```python
from build123d import *

# Parameters (mm, degrees)
SKETCH_1_R          = 1.55
SKETCH_1_R_2        = 6
EXTRUDE_1_DEPTH     = 7
CUT_EXTRUDE_START   = -2
CUT_EXTRUDE_3_DEPTH = 2
SKETCH_4_R          = 2.5
CUT_EXTRUDE_4_DEPTH = 3
CUT_EXTRUDE_5_DEPTH = 5
CUT_EXTRUDE_6_DEPTH = 2
SKETCH_7_W          = 5
SKETCH_7_H          = 3
CUT_EXTRUDE_7_DEPTH = 2


with BuildPart() as part:
    # 草图1 → 凸台-拉伸1 (new body)
    with BuildSketch(Plane.XY):
        with BuildLine():
            Line((0, 3), (73.66, 3))
            Line((73.66, 3), (133.66, 3))
            ThreePointArc((133.66, 3), (135.781320344, 2.121320344), (136.66, 0))
            Line((136.66, 0), (136.66, -21.844))
            Line((136.66, -21.844), (136.66, -43.688))
            ThreePointArc((136.66, -43.688), (135.781320344, -45.809320344), (133.66, -46.688))
            Line((133.66, -46.688), (73.66, -46.688))
            Line((73.66, -46.688), (0, -46.688))
            ThreePointArc((0, -46.688), (-2.121320344, -45.809320344), (-3, -43.688))
            Line((-3, -43.688), (-3, 0))
            ThreePointArc((-3, 0), (-2.121320344, 2.121320344), (0, 3))
        make_face()
        Circle(SKETCH_1_R, mode=Mode.SUBTRACT)
        with Locations((73.66, 0)):
            Circle(SKETCH_1_R, mode=Mode.SUBTRACT)
        with Locations((0, -43.688)):
            Circle(SKETCH_1_R, mode=Mode.SUBTRACT)
        with Locations((73.66, -43.688)):
            Circle(SKETCH_1_R, mode=Mode.SUBTRACT)
        with Locations((106.66, -21.844)):
            Circle(SKETCH_1_R_2, mode=Mode.SUBTRACT)
        with Locations((91.16, -6.344)):
            Circle(SKETCH_1_R, mode=Mode.SUBTRACT)
        with Locations(Location((91.16, -37.344, 0), (0, 0, 180))):
            Circle(SKETCH_1_R, mode=Mode.SUBTRACT)
        with Locations((122.16, -37.344)):
            Circle(SKETCH_1_R, mode=Mode.SUBTRACT)
        with Locations(Location((122.16, -6.344, 0), (0, 0, 180))):
            Circle(SKETCH_1_R, mode=Mode.SUBTRACT)
        with Locations((99.942485579, -15.126485579)):
            Circle(SKETCH_1_R, mode=Mode.SUBTRACT)
        with Locations((113.377514421, -15.126485579)):
            Circle(SKETCH_1_R, mode=Mode.SUBTRACT)
        with Locations((113.377514421, -28.561514421)):
            Circle(SKETCH_1_R, mode=Mode.SUBTRACT)
        with Locations((99.942485579, -28.561514421)):
            Circle(SKETCH_1_R, mode=Mode.SUBTRACT)
        with BuildLine():
            Line((11.83, -15.844), (11.83, -4.844))
            ThreePointArc((11.83, -4.844), (12.708679656, -2.722679656), (14.83, -1.844))
            Line((14.83, -1.844), (36.83, -1.844))
            Line((36.83, -1.844), (58.83, -1.844))
            ThreePointArc((58.83, -1.844), (60.951320344, -2.722679656), (61.83, -4.844))
            Line((61.83, -4.844), (61.83, -15.844))
            ThreePointArc((61.83, -15.844), (60.951320344, -17.965320344), (58.83, -18.844))
            Line((58.83, -18.844), (36.83, -18.844))
            Line((36.83, -18.844), (14.83, -18.844))
            ThreePointArc((14.83, -18.844), (12.708679656, -17.965320344), (11.83, -15.844))
        make_face(mode=Mode.SUBTRACT)
        with BuildLine():
            Line((36.83, -41.844), (58.83, -41.844))
            ThreePointArc((58.83, -41.844), (60.951320344, -40.965320344), (61.83, -38.844))
            Line((61.83, -38.844), (61.83, -27.844))
            ThreePointArc((61.83, -27.844), (60.951320344, -25.722679656), (58.83, -24.844))
            Line((58.83, -24.844), (36.83, -24.844))
            Line((36.83, -24.844), (14.83, -24.844))
            ThreePointArc((14.83, -24.844), (12.708679656, -25.722679656), (11.83, -27.844))
            Line((11.83, -27.844), (11.83, -38.844))
            ThreePointArc((11.83, -38.844), (12.708679656, -40.965320344), (14.83, -41.844))
            Line((14.83, -41.844), (36.83, -41.844))
        make_face(mode=Mode.SUBTRACT)
    extrude(amount=EXTRUDE_1_DEPTH)

    # 草图2 → 切除-拉伸3 (cut)
    with BuildSketch(Plane.XY.offset(7).offset(CUT_EXTRUDE_START)):
        with BuildLine():
            Line((1.933137513, -8), (11.83, -8))
            Line((11.83, -8), (11.83, -15.844))
            ThreePointArc((11.83, -15.844), (12.708679656, -17.965320344), (14.83, -18.844))
            Line((14.83, -18.844), (14.83, -23))
            Line((14.83, -23), (14.83, -24.844))
            ThreePointArc((14.83, -24.844), (12.708679656, -25.722679656), (11.83, -27.844))
            Line((11.83, -27.844), (11.83, -35.779934467))
            Line((11.83, -35.779934467), (1.933137513, -35.779934467))
            Line((1.933137513, -35.779934467), (-3, -35.779934467))
            Line((-3, -35.779934467), (-3, -23))
            Line((-3, -23), (-3, -8))
            Line((-3, -8), (1.933137513, -8))
        make_face()
        Polygon((69.66, -21.844), (69.66, 3), (67.66, 3), (58.66, 3), (58.66, -21.889967233), (58.66, -46.688), (67.66, -46.688), (69.66, -46.688), align=None)
    extrude(amount=CUT_EXTRUDE_3_DEPTH, mode=Mode.SUBTRACT)

    # 草图4 → 切除-拉伸4 (cut)
    with BuildSketch(Plane(origin=(0, 0, 0), x_dir=(-1, 0, 0), z_dir=(0, 0, -1))):
        with Locations((-73.66, 0)):
            Circle(SKETCH_4_R)
        with Locations((-73.66, -43.688)):
            Circle(SKETCH_4_R)
        Circle(SKETCH_4_R)
        with Locations((0, -43.688)):
            Circle(SKETCH_4_R)
    extrude(amount=-CUT_EXTRUDE_4_DEPTH, mode=Mode.SUBTRACT)

    # 草图5 → 切除-拉伸5 (cut)
    with BuildSketch(Plane(origin=(0, 0, 0), x_dir=(-1, 0, 0), z_dir=(0, 0, -1))):
        with BuildLine():
            Line((-85.41, -3.594), (-81.41, -3.594))
            ThreePointArc((-81.41, -3.594), (-79.995786438, -4.179786438), (-79.41, -5.594))
            Line((-79.41, -5.594), (-79.41, -37.094))
            Line((-79.41, -37.094), (-79.41, -38.094))
            ThreePointArc((-79.41, -38.094), (-79.995786438, -39.508213562), (-81.41, -40.094))
            Line((-81.41, -40.094), (-85.41, -40.094))
            ThreePointArc((-85.41, -40.094), (-86.288679656, -42.215320344), (-88.41, -43.094))
            Line((-88.41, -43.094), (-124.91, -43.094))
            ThreePointArc((-124.91, -43.094), (-127.031320344, -42.215320344), (-127.91, -40.094))
            Line((-127.91, -40.094), (-127.91, -3.594))
            ThreePointArc((-127.91, -3.594), (-127.031320344, -1.472679656), (-124.91, -0.594))
            Line((-124.91, -0.594), (-88.41, -0.594))
            ThreePointArc((-88.41, -0.594), (-86.288679656, -1.472679656), (-85.41, -3.594))
        make_face()
    extrude(amount=-CUT_EXTRUDE_5_DEPTH, mode=Mode.SUBTRACT)

    # 草图6 → 切除-拉伸6 (cut)
    with BuildSketch(Plane(origin=(0, 0, 5), x_dir=(-1, 0, 0), z_dir=(0, 0, -1))):
        with BuildLine():
            Line((-82.66, -31.344), (-82.66, -38.344))
            ThreePointArc((-82.66, -38.344), (-81.16, -39.844), (-79.66, -38.344))
            Line((-79.66, -38.344), (-79.66, -31.344))
            ThreePointArc((-79.66, -31.344), (-81.16, -29.844), (-82.66, -31.344))
        make_face()
    extrude(amount=-CUT_EXTRUDE_6_DEPTH, mode=Mode.SUBTRACT)

    # 草图7 → 切除-拉伸7 (cut)
    with BuildSketch(Plane.XY.offset(7)):
        with Locations((72.16, -32.688)):
            Rectangle(SKETCH_7_W, SKETCH_7_H)
    extrude(amount=-CUT_EXTRUDE_7_DEPTH, mode=Mode.SUBTRACT)


solid = part.part
```
The listing builds one solid part. Answer for the finished solid, in the listing's coordinates (mm). A direction names the side the tool comes from. Give positions to 0.01 mm unless a question says otherwise; leave off trailing zeros. Order: outer loops, then holes, each group sorted by start corner. A loop starts at its lowest first (then second) coordinate and runs counter-clockwise, first axis right, second up. Notation, with made-up numbers: (59.25, 53.5) -> (103.25, 53.5) arc R19 cw to (103.25, 71.5) -> close; hole circle Ø10 at (33.5, -5). An arc over 180 degrees is marked (long way). Answer as a JSON object with one key per item and string values. Group by question number.
Item 1: The part is cut by section A-A on x = 52. Write down the section's boundary in (y, z), and give its area (3 significant figures).
Item 2: The part is cut by section D-D on x = 108. Write down the section's boundary in (y, z).
Item 3: A tool of negligible diameter and unlimited length cuts with its end or side. For faces 1 (the flat face through (4, -22, 5)), 2 (the cylindrical face through (0.54, -46.13, 1.48)), 3 (the flat face through (66, 3, 3)), 4 (the cylindrical face through (60.975, -17.942, 2.465)), from which of +Z, -Z, +X, -X, +Y, -Y can it reach the whole face along a straight path? Write none if from no direction.
Item 4: Flat-ended cylindrical pins translate along their axes: pin 1 (4 mm diameter, centred on x = 99.94, y = -15.13, fed in from -Z); pin 2 (4 mm diameter, centred on x = 113.38, y = -28.56, fed in from +Z); pin 3 (4 mm diameter, centred on x = 0, y = 0, fed in from -Z). Find the tip coordinate at first contact, or state that the pin passes through.
Item 5: Determine the mould class of faces 5 (the flat face through (68, -21, 0)), 6 (the cylindrical face through (-2.1, -45.83, 3.45)), 7 (the cylindrical face through (60.975, -25.746, 2.465)) for opening direction Y: pulls with the +Y half, pulls with the -Y half, needs draft (parallel to the pull), parting line crosses it, or undercut.
Item 6: Consider L1, parallel to Y at x = 73.66, z = 0.75; L2, parallel to Y at x = 40, z = 3.25; L3, parallel to X at y = -34, z = 2.25. Determine where each line is inside the solid, lowest interval first. Write a range as from..to.
Item 7: The part is cut by section C-C on z = 1.5. Give the number of separate pieces and of enclosed holes in the cut face, and give its area (3 significant figures).
Item 8: The part is cut by section B-B on x = 91.16. Write down the section's boundary in (y, z), and give its area (3 significant figures).
Result set:
{
 "1": {"outline": "(-46.69, 0) -> (-41.84, 0) -> (-41.84, 7) -> (-46.69, 7) -> close; (-24.84, 0) -> (-18.84, 0) -> (-18.84, 7) -> (-24.84, 7) -> close; (-1.84, 0) -> (3, 0) -> (3, 7) -> (-1.84, 7) -> close", "area": "110 mm²"},
 "2": {"outline": "(-46.69, 0) -> (-43.09, 0) -> (-43.09, 5) -> (-27.69, 5) -> (-27.69, 7) -> (-46.69, 7) -> close; (-16, 5) -> (-0.59, 5) -> (-0.59, 0) -> (3, 0) -> (3, 7) -> (-16, 7) -> close"},
 "3": {"face 1": "+Z, -X", "face 2": "-Z", "face 3": "+Z, -Z, +X, -X, +Y", "face 4": "+Z, -Z"},
 "4": {"pin 1": "z = 5", "pin 2": "z = 7", "pin 3": "z = 3"},
 "5": {"face 5": "needs draft", "face 6": "pulls with the -Y half", "face 7": "undercut"},
 "6": {"L1": "-46.69..-46.19, -41.19..-2.5, 2.5..3", "L2": "-46.69..-41.84, -24.84..-18.84, -1.84..3", "L3": "-3..11.83, 61.83..79.41, 127.91..136.66"},
 "7": {"separate pieces": "1", "enclosed holes": "7", "area": "3,150 mm²"},
 "8": {"outline": "(-46.69, 0) -> (-43.09, 0) -> (-43.09, 5) -> (-38.89, 5) -> (-38.89, 7) -> (-46.69, 7) -> close; (-35.79, 5) -> (-7.89, 5) -> (-7.89, 7) -> (-35.79, 7) -> close; (-4.79, 5) -> (-0.59, 5) -> (-0.59, 0) -> (3, 0) -> (3, 7) -> (-4.79, 7) -> close", "area": "123 mm²"}
}
